Autodesk Fusion 360 part; units mm, degrees
sketch "sketch 234" plane through (0, 0, 0) normal (0, 1, 0) x (1, 0, 0)
  line L0 (-43, -28.5) -> (43, -28.5)
  line L1 (43, -28.5) -> (43, 28.5)
  line L2 (43, 28.5) -> (-43, 28.5)
  line L3 (-43, 28.5) -> (-43, -28.5)
  line L4 (0, -28.5) -> (0, 0) construction
  line L5 (0, 0) -> (43, 0) construction
  circle A0 centre (-39, -24.5) radius 1.5
  circle A1 centre (-15, -15) radius 1.5
  line L6 (-15, -15) -> (15, -15) construction
  circle A2 centre (15, -15) radius 1.5
  line L7 (-15, -15) -> (-15, 15) construction
  circle A3 centre (-15, 15) radius 1.5
  line L8 (15, -15) -> (15, 15) construction
  line L9 (15, 15) -> (-15, 15) construction
  circle A4 centre (15, 15) radius 1.5
  line L10 (0, 15) -> (0, 0) construction
  line L11 (-15, 0) -> (0, 0) construction
  line L12 (44.5, 30) -> (-44.5, 30)
  line L13 (-44.5, 30) -> (-44.5, -30)
  line L14 (-44.5, -30) -> (44.5, -30)
  line L15 (44.5, -30) -> (44.5, 30)
  dimension "d6" = 86
  dimension "d7" = 57
  dimension "d8" = 3
  dimension "d9" = 4
  dimension "d10" = 4
  dimension "d11" = 3
  dimension "d12" = 3
  dimension "d13" = 30
  dimension "d14" = 30
  dimension "d15" = 3
  dimension "d16" = 3
  dimension "d33" = 0
  dimension "d34" = 0
  dimension "d35" = 0
  dimension "d36" = 0
  dimension "d79" = 0
  dimension "d80" = 0
  dimension "d81" = 0
  dimension "d82" = 0
  dimension "d97" = 1.5
extrude "Extrude1" add sketch "sketch 234" against normal blind 14 from surface at 7 contours L12 L13 L14 L15
fillet "Fillet2" radius 2.5 4 edges at (43, 0, 28.5) (43, 0, -28.5) (-43, 0, 28.5) (-43, 0, -28.5)
fillet "Fillet2" radius 4 4 edges at (-44.5, 0, -30) (-44.5, 0, 30) (44.5, 0, 30) (44.5, 0, -30)
sketch "sketch 592" plane through (44.5, 0, 0) normal (1, 0, 0) x (0, 1, 0)
  line L0 (7, 26) -> (7, -26)
  line L1 (7, 26) -> (1, 26)
  line L2 (1, 26) -> (1, -26)
  line L3 (1, -26) -> (7, -26)
  dimension "d122" = 6
extrude "Extrude4" cut sketch "sketch 592" against normal blind 3
equation "d6 = boxWidth"
equation "d7 = boxHeight"
equation "d97 = thickness"
equation "d138 = boxWidth + ( thickness * 2 )"
equation "d139 = boxHeight + ( thickness * 2 )"
equation "d175 = thickness"
equation "d200 = boxHeight / 2"
Design review of the part built by this model. Coordinates are the model's own, in mm. A direction names the side the tool comes from. Round coordinates to 2 decimals unless told otherwise and drop trailing zeros. Loops run counter-clockwise (first coordinate to the right, second up) from the corner with the lowest first, then second, coordinate; pieces in that order, holes last. Notation, with made-up numbers: (9.5, 31.25) - (42.5, 31.25) arc R25 ccw to (42.5, 67.25) - close; hole circle Ø5 at (62, -23.5). An arc over 180 degrees is marked (long way). One line per item, written item: value. Start each with the question number.
1) Draft analysis for pull direction Z (two halves, no side actions). For faces 3 (the flat face through (43, -3, 0)), 4 (the flat face through (-43, 0, 0)), 5 (the flat face through (-13, -7, -29)), 6 (the cylindrical face through (-43.297, -0.098, 28.859)), state which applies: +Z half, -Z half, draft (parallel to the pull), parting line (faces both ways), or undercut.
2) Consider section A-A on y = -4.25. Give the boundary of the cut face in (x, z).
3) Consider section C-C on x = 5. Give the boundary of the cut face in (y, z).
4) Consider section B-B on z = 2. Give the boundary of the cut face in (x, y), then the cut area to 3 significant figures.
5) For faces 1 (the flat face through (1, 0, -28.5)), 2 (the flat face through (-44.5, 0, 0)), list the 3-axis set-ups (+Z, -Z, +X, -X, +Y, -Y) from which the entire face can be reached by the end or side of a thin tool; tool diameter is ignored.
6) Insertion check: pin 1 Ø0.8 at (x, y) = (44, 3) entering from -Z; pin 2 Ø1.6 at (x, y) = (44, 5) entering from +Z. Each pin has a flat end and moves straight along its axis. Give the tip position at first contact, or say it passes through.
7) To check wall thickness, follow L1, parallel to Z at x = -26.5, y = -5; L2, parallel to X at y = -4.5, z = -23.5; L3, parallel to X at y = 5, z = -22. State the ranges of each line that lie inside material, in increasing order. Write a range as from..to.
8) Consider section D-D on y = 4.5. Give the boundary of the cut face in (x, z).
Reported:
1. face 3: undercut
1. face 4: undercut
1. face 5: draft
1. face 6: +Z half
2. outline: (-44.5, -26) arc R4 ccw to (-40.5, -30) - (40.5, -30) arc R4 ccw to (44.5, -26) - (44.5, 26) arc R4 ccw to (40.5, 30) - (-40.5, 30) arc R4 ccw to (-44.5, 26) - close; hole (-43, -26) arc R2.5 ccw to (-40.5, -28.5) - (40.5, -28.5) arc R2.5 ccw to (43, -26) - (43, 26) arc R2.5 ccw to (40.5, 28.5) - (-40.5, 28.5) arc R2.5 ccw to (-43, 26) - close
3. outline: (-7, -30) - (7, -30) - (7, -28.5) - (-7, -28.5) - close; (-7, 28.5) - (7, 28.5) - (7, 30) - (-7, 30) - close
4. outline: (-44.5, -7) - (-43, -7) - (-43, 7) - (-44.5, 7) - close; (43, -7) - (44.5, -7) - (44.5, 1) - (43, 1) - close
4. area: 33.0 mm^2
5. face 1: +Y, -Y
5. face 2: +Z, -Z, -X, +Y, -Y
6. pin 1: stops at z = -28.53
6. pin 2: stops at z = 28.95
7. L1: z = -30..-28.5, 28.5..30
7. L2: x = -44.5..-43, 43..44.5
7. L3: x = -44.5..-43
8. outline: (-44.5, -26) arc R4 ccw to (-40.5, -30) - (40.5, -30) arc R4 ccw to (44.5, -26) - (43, -26) arc R2.5 cw to (40.5, -28.5) - (-40.5, -28.5) arc R2.5 cw to (-43, -26) - (-43, 26) arc R2.5 cw to (-40.5, 28.5) - (40.5, 28.5) arc R2.5 cw to (43, 26) - (44.5, 26) arc R4 ccw to (40.5, 30) - (-40.5, 30) arc R4 ccw to (-44.5, 26) - close
